Design review of the part shown in the three views and the two pictorial views. Dimensions are in mm from the part's minimum x, y and z. A direction names the side the tool comes from. Round coordinates to 2 decimals unless told otherwise and drop trailing zeros. Order: outer loops, then holes, each group sorted by start corner. A loop starts at its lowest first (then second) coordinate and runs counter-clockwise, first axis right, second up.
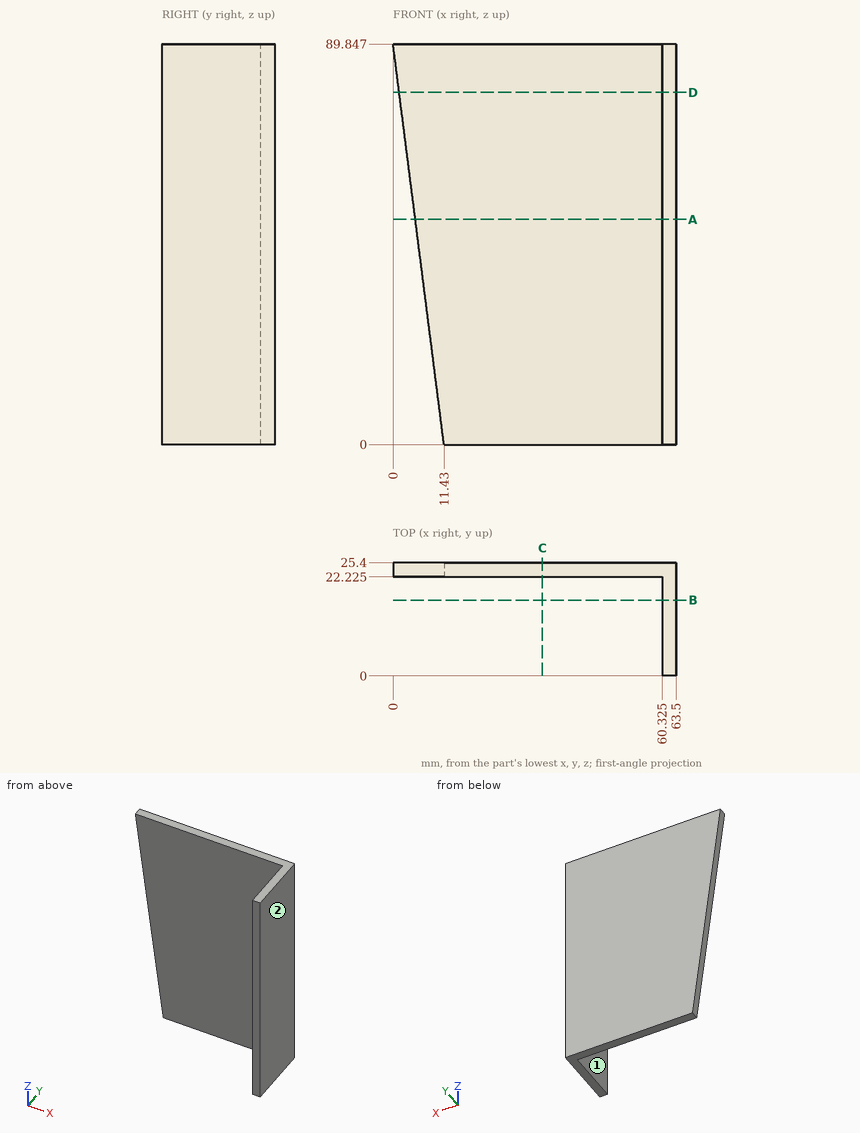
1) Take a section at D-D on z = 79. Give the boundary of the cut face in (x, y) (3 decimals).
Results:
outline: (1.38, 22.225) - (60.325, 22.225) - (60.325, 0) - (63.5, 0) - (63.5, 25.4) - (1.38, 25.4) - close
2) To check wall thickness, follow line 1 along X through (y, z) = (15.25, 44) (3 decimals); line 2 along Y through (x, z) = (58, 27) (3 decimals); line 3 along X through (y, z) = (23, 44). State the ranges of each line that lie inside material, in increasing order.
Results:
line 1: x = 60.325 to 63.5
line 2: y = 22.225 to 25.4
line 3: x = 5.83 to 63.5
3) For the marked faces 1 and 2, list the 3-axis set-ups (+Z, -Z, +X, -X, +Y, -Y) from which the entire face can be reached by the end or side of a thin tool; tool diameter is ignored.
Results:
face 1: +Z, -Z, -X, -Y
face 2: +Z, -Z, +X, +Y, -Y
4) Clearance check with flat-ended pins moving along their axes: P1, Ø18, axis at x = 19, z = 27.5, coming from the -Y side (3 decimals); P2, Ø6, axis at y = 6.5, z = 43.5, coming from the -X side (3 decimals). State where each tip first meets the part, or that it passes through.
Results:
P1: stops at y = 22.225
P2: stops at x = 60.325
5) Take a section at A-A on z = 50.5. Give the boundary of the cut face in (x, y) (1 decimal).
Results:
outline: (5, 22.2) - (60.3, 22.2) - (60.3, 0) - (63.5, 0) - (63.5, 25.4) - (5, 25.4) - close
6) Take a section at C-C on x = 33.5. Give the boundary of the cut face in (y, z) (3 decimals), plus the area to 3 significant figures.
Results:
outline: (22.225, 0) - (25.4, 0) - (25.4, 89.847) - (22.225, 89.847) - close
area: 285 mm2
7) Take a section at B-B on y = 17. Give the boundary of the cut face in (x, z) (3 decimals).
Results:
outline: (60.325, 0) - (63.5, 0) - (63.5, 89.847) - (60.325, 89.847) - close
